Part model, mm, in its own coordinate system. A direction names the side the tool comes from. Coordinates: 2 decimals unless noted, no trailing zeros. Write each loop counter-clockwise with the first axis right and the second up, starting at its lowest first coordinate (ties: lowest second). Pieces come first, ordered by that corner, then holes. Notation, with made-up numbers: (-1.5, -34) -> (45.5, -34) arc R22 cw to (45.5, -28) -> close; hole circle Ø4 at (-36, -19). An arc over 180 degrees is marked (long way). Write item = value, one per line.
from build123d import *

# Parameters (mm, degrees)
LINEAR_AUSTRAGEN_D_NN1_DEPTH    = 15
AUFSATZ_LINEAR_AUSTRAGEN1_DEPTH = 1.2
SKIZZE3_R                       = 5.25
SCHNITT_LINEAR_AUSTRAGEN1_DEPTH = 1.2
SKIZZE4_W                       = 4.4
SKIZZE4_H                       = 4.707579954
SCHNITT_LINEAR_AUSTRAGEN2_DEPTH = 1.2


with BuildPart() as part:
    # Skizze1 → Linear-Austragen-Dünn1 (new body)
    with BuildSketch(Plane.XY):
        Polygon((0, -20), (17.320508076, -10), (17.320508076, 10), (0, 20), (-17.320508076, 10), (-17.320508076, -10), align=None)
        Polygon((0, -18.614359354), (16.120508076, -9.307179677), (16.120508076, 9.307179677), (0, 18.614359354), (-16.120508076, 9.307179677), (-16.120508076, -9.307179677), align=None, mode=Mode.SUBTRACT)
    extrude(amount=LINEAR_AUSTRAGEN_D_NN1_DEPTH)

    # Skizze2 → Aufsatz-Linear austragen1 (add)
    with BuildSketch(Plane(origin=(0, 0, 0), x_dir=(-1, 0, 0), z_dir=(0, 0, -1))):
        Polygon((-16.120508076, -9.307179677), (-16.120508076, 9.307179677), (0, 18.614359354), (16.120508076, 9.307179677), (16.120508076, -9.307179677), (0, -18.614359354), align=None)
    extrude(amount=-AUFSATZ_LINEAR_AUSTRAGEN1_DEPTH)

    # Skizze3 → Schnitt-Linear austragen1 (cut)
    with BuildSketch(Plane.XY.offset(1.2)):
        with Locations((0, -11.695345197)):
            Circle(SKIZZE3_R)
    extrude(amount=-SCHNITT_LINEAR_AUSTRAGEN1_DEPTH, mode=Mode.SUBTRACT)

    # Skizze4 → Schnitt-Linear austragen2 (cut)
    with BuildSketch(Plane.XY.offset(1.2)):
        with Locations((0, -6.653789977)):
            Rectangle(SKIZZE4_W, SKIZZE4_H)
    extrude(amount=-SCHNITT_LINEAR_AUSTRAGEN2_DEPTH, mode=Mode.SUBTRACT)


solid = part.part
Q1. Saw through at B-B on z = 7. Give the cut face in (x, y), and give its area (3 significant figures).
Model answer:
outline = (-17.32, -10) -> (0, -20) -> (17.32, -10) -> (17.32, 10) -> (0, 20) -> (-17.32, 10) -> close; hole (-16.12, -9.31) -> (0, -18.61) -> (16.12, -9.31) -> (16.12, 9.31) -> (0, 18.61) -> (-16.12, 9.31) -> close
area = 139 mm²
Q2. Probe line 1 (X direction, y = -1, z = 9); line 2 (Y direction, x = 0, z = 0.85); line 3 (Z direction, x = -1.5, y = 4.5). List the from-to ranges inside material, lowest first. Write a range as from..to.
Model answer:
line_1 = -17.32..-16.12, 16.12..17.32
line_2 = -20..-16.95, -4.3..20
line_3 = 0..1.2
Q3. Saw through at D-D on y = 1. Give the cut face in (x, z), and give its area (3 significant figures).
Model answer:
outline = (-17.32, 0) -> (17.32, 0) -> (17.32, 15) -> (16.12, 15) -> (16.12, 1.2) -> (-16.12, 1.2) -> (-16.12, 15) -> (-17.32, 15) -> close
area = 74.7 mm²
Q4. Mould opens along X. For faces 1 (the face through (8.54, -15.07, 7.4)), 2 (the face through (-7.947, 14.026, 8.003)), 3 (the face through (0, 0, 0)), 4 (the face through (-8.54, 15.07, 7.4)) say: released by +X, released by -X, zero draft, split by the parting line, or undercut.
Model answer:
face_1 = released by +X
face_2 = undercut
face_3 = zero draft
face_4 = released by -X
Q5. Which spindle directions (+Z, -Z, +X, -X, +Y, -Y) get a long thin tool onto all of the face, cutting with end or side? Do faces 5 (the face through (16.121, 0, 8)), 6 (the face through (-2.2, -6, 1)), 7 (the face through (8.78, 14.93, 7.4)). Say none if no direction does.
Model answer:
face_5 = +Z
face_6 = +Z, -Z
face_7 = +Z, -Z, +X, +Y
Q6. Saw through at A-A on y = -6. Give the cut face in (x, z), and give its area (3 significant figures).
Model answer:
outline = (-17.32, 0) -> (-2.2, 0) -> (-2.2, 1.2) -> (-16.12, 1.2) -> (-16.12, 15) -> (-17.32, 15) -> close; (2.2, 0) -> (17.32, 0) -> (17.32, 15) -> (16.12, 15) -> (16.12, 1.2) -> (2.2, 1.2) -> close
area = 69.4 mm²
Q7. Pin check, flat tips, straight feed: pin 1 (2 mm diameter, centred on x = 9, z = 11.5, fed in from -Y); pin 2 (1.5 mm diameter, centred on x = 1, z = 6, fed in from +Y); pin 3 (5 mm diameter, centred on x = 5, z = 4, fed in from +Y); pin 4 (1 mm diameter, centred on x = -3, y = 2.5, fed in from -Z). Stop position of each tip, or through.
Model answer:
pin_1 = -15.38
pin_2 = 19.86
pin_3 = 18.56
pin_4 = 0
Q8. Saw through at C-C on x = -1.5. Give the cut face in (y, z).
Model answer:
outline = (-19.13, 0) -> (-16.73, 0) -> (-16.73, 1.2) -> (-17.75, 1.2) -> (-17.75, 15) -> (-19.13, 15) -> close; (-4.3, 0) -> (19.13, 0) -> (19.13, 15) -> (17.75, 15) -> (17.75, 1.2) -> (-4.3, 1.2) -> close
